```python
from build123d import *

# Parameters (mm, degrees)
SKETCH3_R           = 1.2573
CUT_EXTRUDE1_DEPTH  = 25.781842813
SKETCH4_R           = 3.175
SKETCH4_R_2         = 1.5875
BOSS_EXTRUDE1_DEPTH = 3.175


with BuildPart() as part:
    # Sketch1 → Revolve1 (revolve)
    with BuildSketch(Plane.XY, mode=Mode.PRIVATE) as revolve1_sk:
        Polygon((17.3789975, 3.175), (17.3789975, 0), (3.5, 0), (3.5, 3.175), (14.2039975, 3.175), align=None)
    revolve(revolve1_sk.sketch.rotate(Axis((0, 0, 0), (0, 1, 0)), 90), axis=Axis((0, 0, 0), (0, 1, 0)))

    # Sketch3 → Cut-Extrude1 (cut, through all)
    with BuildSketch(Plane(origin=(0, 3.175, 0), x_dir=(1, 0, 0), z_dir=(0, 1, 0))):
        with Locations(Location((0, -9.5, 0), (0, 0, 270))):
            Circle(SKETCH3_R)
        with Locations(Location((-8.000000002, 0, 0), (0, 0, 270))):
            Circle(SKETCH3_R)
        with Locations(Location((0, 9.5, 0), (0, 0, 270))):
            Circle(SKETCH3_R)
        with Locations(Location((8.000000002, 0, 0), (0, 0, 270))):
            Circle(SKETCH3_R)
    extrude(amount=-CUT_EXTRUDE1_DEPTH, mode=Mode.SUBTRACT)

    # Sketch4 → Boss-Extrude1 (add)
    # profile 1 of 6: a face of its own
    with BuildSketch(Plane(origin=(0, 0, 0), x_dir=(1, 0, 0), z_dir=(0, 1, 0))):
        with Locations((-14.533871013, 14.533871013)):
            Circle(SKETCH4_R)
        with Locations(Location((-14.533871013, 14.533871013, 0), (0, 0, 270))):
            Circle(SKETCH4_R_2, mode=Mode.SUBTRACT)
    # profile 2 of 6: a face of its own
    with BuildSketch(Plane(origin=(0, 0, 0), x_dir=(1, 0, 0), z_dir=(0, 1, 0))):
        with BuildLine():
            ThreePointArc((-12.288807066, 12.288806898), (-11.109708346, 13.364278303), (-9.836925233, 14.327053293))
            Line((-9.836925233, 14.327053293), (-12.288806982, 16.778935043))
            ThreePointArc((-12.288806982, 16.778935043), (-11.600553497, 15.74889091), (-11.358871013, 14.533871013))
            ThreePointArc((-11.358871013, 14.533871013), (-11.60055352, 13.31885106), (-12.288807066, 12.288806899))
        make_face()
    # profile 3 of 6: a face of its own
    with BuildSketch(Plane(origin=(0, 0, 0), x_dir=(1, 0, 0), z_dir=(0, 1, 0))):
        with BuildLine():
            ThreePointArc((-14.327053293, 9.836925233), (-13.364278379, 11.109708255), (-12.288807066, 12.288806898))
            ThreePointArc((-12.288807066, 12.288806899), (-14.533871072, 11.358871013), (-16.778935043, 12.288806982))
            Line((-16.778935043, 12.288806982), (-14.327053293, 9.836925233))
        make_face()
    # profile 4 of 6: a face of its own
    with BuildSketch(Plane(origin=(0, 0, 0), x_dir=(1, 0, 0), z_dir=(0, 1, 0))):
        with Locations((14.533871013, -14.533871013)):
            Circle(SKETCH4_R)
        with Locations(Location((14.533871013, -14.533871013, 0), (0, 0, 270))):
            Circle(SKETCH4_R_2, mode=Mode.SUBTRACT)
    # profile 5 of 6: a face of its own
    with BuildSketch(Plane(origin=(0, 0, 0), x_dir=(1, 0, 0), z_dir=(0, 1, 0))):
        with BuildLine():
            ThreePointArc((12.288806982, -16.778935043), (11.358871013, -14.533870968), (12.288807046, -12.288806919))
            ThreePointArc((12.288807046, -12.288806919), (11.109708335, -13.364278313), (9.836925233, -14.327053293))
            Line((9.836925233, -14.327053293), (12.288806982, -16.778935043))
        make_face()
    # profile 6 of 6: a face of its own
    with BuildSketch(Plane(origin=(0, 0, 0), x_dir=(1, 0, 0), z_dir=(0, 1, 0))):
        with BuildLine():
            ThreePointArc((12.288807046, -12.288806919), (14.533871058, -11.358871013), (16.778935043, -12.288806982))
            Line((16.778935043, -12.288806982), (14.327053293, -9.836925233))
            ThreePointArc((14.327053293, -9.836925233), (13.36427837, -11.109708266), (12.288807046, -12.288806919))
        make_face()
    extrude(amount=BOSS_EXTRUDE1_DEPTH)


solid = part.part
```
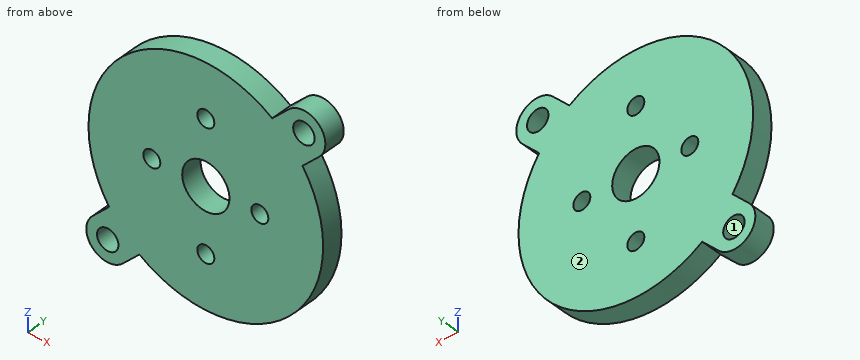
Geometry check sheet. Reference: the model listing, model coordinates, mm. Face numbers are marked on the shaded views. Coordinates: 2 decimals unless noted, no trailing zeros. Order: outer loops, then holes, each group sorted by start corner. A loop starts at its lowest first (then second) coordinate and runs counter-clockwise, first axis right, second up. Notation, with made-up numbers: (-20, -21) - (3, -21) arc R24 cw to (3, -7) - close; hole circle Ø6 at (21, 68.25). An arc over 180 degrees is marked (long way). Answer as a JSON object with one key per item and string values. Group by question number.
Item 1: Sectioned sample at B-B, the plane x = 0. Record the cut outline in (y, z) (3 decimals), and give its area (3 significant figures).
Item 2: Sectioned sample at C-C, the plane x = -8. Record the cut outline in (y, z) (3 decimals), and give its area (3 significant figures).
Item 3: Sectioned sample at D-D, the plane y = 0.6. Give the number of separate pieces and of enclosed holes in the cut face, and give its area (3 significant figures).
Item 4: Draft check along Z on the marked faces 1 and 2. Enter one of: +Z half, -Z half, draft (parallel to the pull), parting line (faces both ways), or undercut.
Item 5: Depth check by flat-ended pin: pin 1 Ø2 at (x, z) = (0, 9.5) entering from +Y; pin 2 Ø1 at (y, z) = (1.5, -10) entering from -X; pin 3 Ø1 at (y, z) = (1.5, -9) entering from -X; pin 4 Ø1.5 at (y, z) = (2, 5.5) entering from -X. Enter the tip coordinate at first touch or a pass-through.
Item 6: Scan lines: probe 1 along X at (y, z) = (0.7, 0); probe 2 along X at (y, z) = (1.7, 15); probe 3 along X at (y, z) = (1.55, 1). Record each from-to range of solid material in increasing order.
Item 7: Sectioned sample at A-A, the plane z = 0. Record the cut outline in (x, y) (3 decimals).
Resolved:
{
 "1": {"outline": "(0, -17.379) - (3.175, -17.379) - (3.175, -10.757) - (0, -10.757) - close; (0, -8.243) - (3.175, -8.243) - (3.175, -3.5) - (0, -3.5) - close; (0, 3.5) - (3.175, 3.5) - (3.175, 8.243) - (0, 8.243) - close; (0, 10.757) - (3.175, 10.757) - (3.175, 17.379) - (0, 17.379) - close", "area": "72.2 mm^2"},
 "2": {"outline": "(0, -15.428) - (3.175, -15.428) - (3.175, -1.257) - (0, -1.257) - close; (0, 1.257) - (3.175, 1.257) - (3.175, 15.428) - (0, 15.428) - close", "area": "90.0 mm^2"},
 "3": {"separate pieces": "1", "enclosed holes": "7", "area": "948 mm^2"},
 "4": {"face 1": "undercut", "face 2": "draft"},
 "5": {"pin 1": "through", "pin 2": "x = -14.99", "pin 3": "x = -15.16", "pin 4": "x = -16.72"},
 "6": {"probe 1": "-17.38 to -9.26, -6.74 to -3.5, 3.5 to 6.74, 9.26 to 17.38", "probe 2": "-8.78 to 8.78, 10.51 to 13.02, 16.05 to 17.67", "probe 3": "-17.35 to -8.76, -7.24 to -3.35, 3.35 to 7.24, 8.76 to 17.35"},
 "7": {"outline": "(-17.379, 0) - (-9.257, 0) - (-9.257, 3.175) - (-17.379, 3.175) - close; (-6.743, 0) - (-3.5, 0) - (-3.5, 3.175) - (-6.743, 3.175) - close; (3.5, 0) - (6.743, 0) - (6.743, 3.175) - (3.5, 3.175) - close; (9.257, 0) - (17.379, 0) - (17.379, 3.175) - (9.257, 3.175) - close"}
}
